The model under review builds one solid part; all positions refer to its coordinate system, in mm. A direction names the side the tool comes from. Coordinates: 2 decimals unless noted, no trailing zeros. Order: outer loops, then holes, each group sorted by start corner. A loop starts at its lowest first (then second) coordinate and runs counter-clockwise, first axis right, second up. Notation, with made-up numbers: (-25.75, 70) - (-13.75, 70) arc R17 ccw to (-13.75, 86) - close; hole circle Ø9 at (-11, -9). An arc over 180 degrees is marked (long way). Answer in a Markdown table with one row per item.
```python
from build123d import *

# Parameters (mm, degrees)
SKETCH1_W                       = 127
SKETCH1_H                       = 25.4
SKETCH1_W_2                     = 25.4
SKETCH1_H_2                     = 50.8
BOSS_EXTRUDE1_DEPTH             = 3.175
F_5_32_0_15625_DIAMETER_HOLE1_D = 3.96875
SKETCH4_W                       = 6.35
SKETCH4_H                       = 76.2
BOSS_EXTRUDE2_DEPTH             = 12.7
FILLET2_R                       = 6.35


with BuildPart() as part:
    # Sketch1 → Boss-Extrude1 (new, symmetric)
    with BuildSketch(Plane(origin=(0, 0, 0), x_dir=(1, 0, 0), z_dir=(0, 1, 0))):
        Polygon((-139.7, -12.7), (-139.7, 12.7), (-139.7, 38.1), (-165.1, 38.1), (-165.1, -38.1), (-139.7, -38.1), align=None)
        with Locations((-76.2, 0)):
            Rectangle(SKETCH1_W, SKETCH1_H)
        with Locations((0, 38.1)):
            Rectangle(SKETCH1_W_2, SKETCH1_H_2)
        with Locations((76.2, 0)):
            Rectangle(SKETCH1_W, SKETCH1_H)
        Rectangle(SKETCH1_W_2, SKETCH1_H)
        with Locations((0, -38.1)):
            Rectangle(SKETCH1_W_2, SKETCH1_H_2)
        Polygon((139.7, 38.1), (139.7, 12.7), (139.7, -12.7), (139.7, -38.1), (165.1, -38.1), (165.1, 38.1), align=None)
    extrude(amount=BOSS_EXTRUDE1_DEPTH, both=True)

    # 5/32 (0.15625) Diameter Hole1 (through all)
    with Locations(Plane(origin=(0, 3.175, 0), x_dir=(1, 0, 0), z_dir=(0, 1, 0))):
        with Locations((0, 25.4), (0, -25.4)):
            Hole(F_5_32_0_15625_DIAMETER_HOLE1_D / 2)

    # Sketch4 → Boss-Extrude2 (add)
    with BuildSketch(Plane(origin=(0, 3.175, 0), x_dir=(1, 0, 0), z_dir=(0, 1, 0))):
        with Locations((161.925, 0)):
            Rectangle(SKETCH4_W, SKETCH4_H)
        with Locations((-161.925, 0)):
            Rectangle(SKETCH4_W, SKETCH4_H)
    extrude(amount=BOSS_EXTRUDE2_DEPTH)

    # Fillet2
    fillet2_edges = [part.edges().sort_by_distance(p)[0] for p in [
        (-139.7, 0, -12.7),
        (-12.7, 0, -12.7),
        (-12.7, 0, -63.5),
        (12.7, 0, -63.5),
        (12.7, 0, -12.7),
        (139.7, 0, -12.7),
        (139.7, 0, -38.1),
        (139.7, 0, 38.1),
        (139.7, 0, 12.7),
        (12.7, 0, 12.7),
        (12.7, 0, 63.5),
        (-12.7, 0, 63.5),
        (-12.7, 0, 12.7),
        (-139.7, 0, 12.7),
        (-139.7, 0, 38.1),
        (-139.7, 0, -38.1),
        (158.75, 3.175, 0),
        (-158.75, 3.175, 0),
    ]]
    fillet(fillet2_edges, radius=FILLET2_R)


solid = part.part
```
Item 1: Tool access review of faces 5 (the face through (-14.51, 0.04, 14.61)), 6 (the face through (141.51, 0.04, -36.19)), 7 (the face through (156.939, 5.085, -0.533)): name each direction out of +Z, -Z, +X, -X, +Y, -Y from which nothing blocks a thin tool from reaching the whole face with its end or side.
Check values:
| item | result |
|---|---|
| face 5 | +Z, +Y, -Y |
| face 6 | -Z, +Y, -Y |
| face 7 | +Z, -Z, +Y |
Item 2: To check wall thickness, follow line 1 (X direction, y = -0.75, z = -25.4); line 2 (Z direction, x = 0, y = 1.5); line 3 (X direction, y = -1.5, z = 20). State the ranges of each line that lie inside material, in increasing order. Write a range as from..to.
Check values:
| item | result |
|---|---|
| line 1 | -165.1..-139.7, -12.7..-1.98, 1.98..12.7, 139.7..165.1 |
| line 2 | -63.5..-27.38, -23.42..23.42, 27.38..63.5 |
| line 3 | -165.1..-139.7, -12.7..12.7, 139.7..165.1 |
Item 3: We need section B-B, the plane z = -46. Write out the cut boundary in (x, y) (3 decimals), then the cut area to 3 significant figures.
Check values:
| item | result |
|---|---|
| outline | (-12.7, -3.175) - (12.7, -3.175) - (12.7, 3.175) - (-12.7, 3.175) - close |
| area | 161 mm^2 |
Item 4: We need section C-C, the plane x = 69.5. Write out the cut boundary in (y, z) (3 decimals).
Check values:
| item | result |
|---|---|
| outline | (-3.175, -12.7) - (3.175, -12.7) - (3.175, 12.7) - (-3.175, 12.7) - close |
Item 5: Mouldability with a two-part tool opening along X and no side actions: class faces 1 (the face through (-165.1, 6, -1)), 2 (the face through (158.75, 13, 1)), 3 (the face through (165.1, 6, 1)), 4 (the face through (0, 0, 63.5)) as +X half, -X half, draft (parallel to the pull), parting line (faces both ways), or undercut.
Check values:
| item | result |
|---|---|
| face 1 | -X half |
| face 2 | undercut |
| face 3 | +X half |
| face 4 | draft |
Item 6: We need section A-A, the plane z = 16. Write out the cut boundary in (x, y) (3 decimals).
Check values:
| item | result |
|---|---|
| outline | (-165.1, -3.175) - (-138.92, -3.175) - (-138.92, 3.175) - (-152.4, 3.175) arc R6.35 cw to (-158.75, 9.525) - (-158.75, 15.875) - (-165.1, 15.875) - close; (-13.48, -3.175) - (13.48, -3.175) - (13.48, 3.175) - (-13.48, 3.175) - close; (138.92, -3.175) - (165.1, -3.175) - (165.1, 15.875) - (158.75, 15.875) - (158.75, 9.525) arc R6.35 cw to (152.4, 3.175) - (138.92, 3.175) - close |
Item 7: Clearance check with flat-ended pins moving along their axes: pin 1 Ø1.5 at (x, y) = (-43, 2) entering from +Z; pin 2 Ø5.5 at (x, y) = (-152.5, 5.5) entering from +Z; pin 3 Ø5 at (y, z) = (0, -43.5) entering from +X; pin 4 Ø5.5 at (x, y) = (154, 9.5) entering from -Z. State where each tip first meets the part, or that it passes through.
Check values:
| item | result |
|---|---|
| pin 1 | z = 12.7 |
| pin 2 | z = 38.1 |
| pin 3 | x = 12.7 |
| pin 4 | through |
